Here's how the part is built. I have some questions about the finished solid (model axes, mm). A direction names the side the tool comes from. Coordinates: 2 decimals unless noted, no trailing zeros. Loops run counter-clockwise (first coordinate to the right, second up) from the corner with the lowest first, then second, coordinate; pieces in that order, holes last. Notation, with made-up numbers: (19, -30) -> (66, -30) arc R29 cw to (66, -10) -> close; hole circle Ø6 at (73, -27.75). An arc over 180 degrees is marked (long way). Answer as a JSON object with one key per item and string values. Group by question number.
1) If we mould it in two halves opening along Z, with no side actions, what happens to faces 1 (the flat face through (-1, 3, -6)), 2 (the cylindrical face through (62.325, 1.479, 108.237)), 3 (the cylindrical face through (48.55, 1.52, 68.16))? For each: +Z half, -Z half, draft (parallel to the pull), parting line (faces both ways), or undercut.
2) I need wall thicknesses on probe 1 along Z at (x, y) = (-31, 1.4); probe 2 along X at (y, z) = (1, -110); probe 3 along Z at (x, y) = (-54, 2.35). Which ranges of each line are inside material? Lowest first, please. Write a range as [from, to].
3) I want a section at C-C (y = 1.55). Count the separate pieces of the cut face and the enclosed holes in it, then the cut area to 3 significant figures.
4) I want a section at A-A (x = 23.5). Write out the boundary of the cut face in (y, z).
5) I want a section at B-B (x = 6.5). Write out the boundary of the cut face in (y, z), then the cut area to 3 significant figures.
6) I'm going to push flat-ended pins straight in: pin 1 (2 mm diameter, centred on x = 14.5, z = 67.27, fed in from +Y); pin 2 (3 mm diameter, centred on x = -34.5, z = 86.5, fed in from -Y); pin 3 (1.6 mm diameter, centred on x = 34.5, y = 1.5, fed in from +Z). Where does each tip first touch, or does it pass through?
7) Which directions (+Z, -Z, +X, -X, +Y, -Y) give clear straight access to the entire face, cutting with the end or side of a thin tool? Please do faces 4 (the cylindrical face through (-62.325, 1.479, 108.237)), 5 (the cylindrical face through (56.1, 1.5, 34.4)), 6 (the cylindrical face through (-41.32, 1.48, 108.24)).
```python
from build123d import *

# Parameters (mm, degrees)
SKETCH1_W           = 180
SKETCH1_H           = 240
BOSS_EXTRUDE1_DEPTH = 3
SKETCH3_R           = 1.55
CUT_EXTRUDE2_DEPTH  = 151.029997001
SKETCH4_R           = 1.6
SKETCH4_R_2         = 1.65
CUT_EXTRUDE3_DEPTH  = 151.029997001
SKETCH5_R           = 1.6
CUT_EXTRUDE4_DEPTH  = 151.029997001
SKETCH6_R           = 1.55
CUT_EXTRUDE5_DEPTH  = 151.029997001
SKETCH7_W           = 25.678556749
SKETCH7_H           = 240
SKETCH7_W_2         = 78.7
SKETCH7_H_2         = 25
CUT_EXTRUDE6_DEPTH  = 151.029997001
SKETCH8_W           = 128.642886502
SKETCH8_H           = 9.657988802
CUT_EXTRUDE7_DEPTH  = 137.184610224
FILLET1_R           = 7


with BuildPart() as part:
    # Sketch1 → Boss-Extrude1 (new body)
    with BuildSketch(Plane(origin=(0, 0, 0), x_dir=(1, 0, 0), z_dir=(0, 1, 0))):
        Rectangle(SKETCH1_W, SKETCH1_H)
    extrude(amount=BOSS_EXTRUDE1_DEPTH)

    # Sketch3 → Cut-Extrude2 (cut, through all)
    with BuildSketch(Plane(origin=(0, 3, 0), x_dir=(1, 0, 0), z_dir=(0, 1, 0))):
        with Locations(Location((14, 110, 0), (0, 0, 270))):
            Circle(SKETCH3_R)
        with Locations(Location((-14, 110, 0), (0, 0, 90))):
            Circle(SKETCH3_R)
    extrude(amount=-CUT_EXTRUDE2_DEPTH, mode=Mode.SUBTRACT)

    # Sketch4 → Cut-Extrude3 (cut, through all)
    with BuildSketch(Plane(origin=(0, 3, 0), x_dir=(1, 0, 0), z_dir=(0, 1, 0))):
        with Locations(Location((-50.5, -32.268683434, 0), (0, 0, 270))):
            Circle(SKETCH4_R)
        with Locations(Location((-50.5, -67.268683434, 0), (0, 0, 270))):
            Circle(SKETCH4_R)
        with Locations(Location((14.5, -32.268683434, 0), (0, 0, 270))):
            Circle(SKETCH4_R_2)
        with Locations(Location((14.5, -67.268683434, 0), (0, 0, 270))):
            Circle(SKETCH4_R_2)
    extrude(amount=-CUT_EXTRUDE3_DEPTH, mode=Mode.SUBTRACT)

    # Sketch5 → Cut-Extrude4 (cut, through all)
    with BuildSketch(Plane(origin=(0, 3, 0), x_dir=(1, 0, 0), z_dir=(0, 1, 0))):
        with Locations(Location((56, 54.660722259, 0), (0, 0, 270))):
            Circle(SKETCH5_R)
        with Locations(Location((56, -18.339277741, 0), (0, 0, 270))):
            Circle(SKETCH5_R)
        with Locations(Location((-56, -18.339277741, 0), (0, 0, 270))):
            Circle(SKETCH5_R)
        with Locations(Location((-56, 54.660722259, 0), (0, 0, 270))):
            Circle(SKETCH5_R)
    extrude(amount=-CUT_EXTRUDE4_DEPTH, mode=Mode.SUBTRACT)

    # Sketch6 → Cut-Extrude5 (cut, through all)
    with BuildSketch(Plane(origin=(0, 3, 0), x_dir=(1, 0, 0), z_dir=(0, 1, 0))):
        with Locations(Location((-54.321443251, -103.342011198, 0), (0, 0, 270))):
            Circle(SKETCH6_R)
        with Locations(Location((54.378556749, -103.342011198, 0), (0, 0, 270))):
            Circle(SKETCH6_R)
        with Locations(Location((-54.321443251, 104.657988802, 0), (0, 0, 270))):
            Circle(SKETCH6_R)
        with Locations(Location((54.378556749, 104.657988802, 0), (0, 0, 270))):
            Circle(SKETCH6_R)
    extrude(amount=-CUT_EXTRUDE5_DEPTH, mode=Mode.SUBTRACT)

    # Sketch7 → Cut-Extrude6 (cut, through all)
    with BuildSketch(Plane(origin=(0, 3, 0), x_dir=(1, 0, 0), z_dir=(0, 1, 0))):
        with BuildLine():
            Line((37.630016224, 79.701073582), (12.399273995, 79.701073582))
            ThreePointArc((12.399273995, 79.701073582), (10.985060433, 80.286860019), (10.399273995, 81.701073582))
            Line((10.399273995, 81.701073582), (10.399273995, 81.912178755))
            ThreePointArc((10.399273995, 81.912178755), (10.985060433, 83.326392317), (12.399273995, 83.912178755))
            Line((12.399273995, 83.912178755), (37.630016224, 83.912178755))
            ThreePointArc((37.630016224, 83.912178755), (39.044229786, 83.326392317), (39.630016224, 81.912178755))
            Line((39.630016224, 81.912178755), (39.630016224, 81.701073582))
            ThreePointArc((39.630016224, 81.701073582), (39.044229786, 80.286860019), (37.630016224, 79.701073582))
        make_face()
        with BuildLine():
            Line((-37.630016224, 83.912178755), (-12.399273995, 83.912178755))
            ThreePointArc((-12.399273995, 83.912178755), (-10.985060433, 83.326392317), (-10.399273995, 81.912178755))
            Line((-10.399273995, 81.912178755), (-10.399273995, 81.701073582))
            ThreePointArc((-10.399273995, 81.701073582), (-10.985060433, 80.286860019), (-12.399273995, 79.701073582))
            Line((-12.399273995, 79.701073582), (-37.630016224, 79.701073582))
            ThreePointArc((-37.630016224, 79.701073582), (-39.044229786, 80.286860019), (-39.630016224, 81.701073582))
            Line((-39.630016224, 81.701073582), (-39.630016224, 81.912178755))
            ThreePointArc((-39.630016224, 81.912178755), (-39.044229786, 83.326392317), (-37.630016224, 83.912178755))
        make_face()
        with Locations((-77.160721626, 0)):
            Rectangle(SKETCH7_W, SKETCH7_H)
        with Locations((0.028556749, -107.5)):
            Rectangle(SKETCH7_W_2, SKETCH7_H_2)
        with Locations((77.160721626, 0)):
            Rectangle(SKETCH7_W, SKETCH7_H)
        with BuildLine():
            Line((29.345445331, -37.30118784), (29.345445331, -65.30118784))
            ThreePointArc((29.345445331, -65.30118784), (30.517018206, -68.129614965), (33.345445331, -69.30118784))
            Line((33.345445331, -69.30118784), (35.345445331, -69.30118784))
            ThreePointArc((35.345445331, -69.30118784), (38.173872456, -68.129614965), (39.345445331, -65.30118784))
            Line((39.345445331, -65.30118784), (39.345445331, -37.30118784))
            ThreePointArc((39.345445331, -37.30118784), (38.173872456, -34.472760715), (35.345445331, -33.30118784))
            Line((35.345445331, -33.30118784), (33.345445331, -33.30118784))
            ThreePointArc((33.345445331, -33.30118784), (30.517018206, -34.472760715), (29.345445331, -37.30118784))
        make_face()
        with BuildLine():
            Line((51.345445331, -33.30118784), (53.345445331, -33.30118784))
            ThreePointArc((53.345445331, -33.30118784), (56.173872456, -34.472760715), (57.345445331, -37.30118784))
            Line((57.345445331, -37.30118784), (57.345445331, -65.30118784))
            ThreePointArc((57.345445331, -65.30118784), (56.173872456, -68.129614965), (53.345445331, -69.30118784))
            Line((53.345445331, -69.30118784), (51.345445331, -69.30118784))
            ThreePointArc((51.345445331, -69.30118784), (48.517018206, -68.129614965), (47.345445331, -65.30118784))
            Line((47.345445331, -65.30118784), (47.345445331, -37.30118784))
            ThreePointArc((47.345445331, -37.30118784), (48.517018206, -34.472760715), (51.345445331, -33.30118784))
        make_face()
        with BuildLine():
            Line((37.630016224, 94.701073582), (12.399273995, 94.701073582))
            ThreePointArc((12.399273995, 94.701073582), (10.985060433, 95.286860019), (10.399273995, 96.701073582))
            Line((10.399273995, 96.701073582), (10.399273995, 96.912178755))
            ThreePointArc((10.399273995, 96.912178755), (10.985060433, 98.326392317), (12.399273995, 98.912178755))
            Line((12.399273995, 98.912178755), (37.630016224, 98.912178755))
            ThreePointArc((37.630016224, 98.912178755), (39.044229786, 98.326392317), (39.630016224, 96.912178755))
            Line((39.630016224, 96.912178755), (39.630016224, 96.701073582))
            ThreePointArc((39.630016224, 96.701073582), (39.044229786, 95.286860019), (37.630016224, 94.701073582))
        make_face()
        with BuildLine():
            Line((-37.630016224, 98.912178755), (-12.399273995, 98.912178755))
            ThreePointArc((-12.399273995, 98.912178755), (-10.985060433, 98.326392317), (-10.399273995, 96.912178755))
            Line((-10.399273995, 96.912178755), (-10.399273995, 96.701073582))
            ThreePointArc((-10.399273995, 96.701073582), (-10.985060433, 95.286860019), (-12.399273995, 94.701073582))
            Line((-12.399273995, 94.701073582), (-37.630016224, 94.701073582))
            ThreePointArc((-37.630016224, 94.701073582), (-39.044229786, 95.286860019), (-39.630016224, 96.701073582))
            Line((-39.630016224, 96.701073582), (-39.630016224, 96.912178755))
            ThreePointArc((-39.630016224, 96.912178755), (-39.044229786, 98.326392317), (-37.630016224, 98.912178755))
        make_face()
    extrude(amount=-CUT_EXTRUDE6_DEPTH, mode=Mode.SUBTRACT)

    # Sketch8 → Cut-Extrude7 (cut, through all)
    with BuildSketch(Plane(origin=(0, 3, 0), x_dir=(1, 0, 0), z_dir=(0, 1, 0))):
        with Locations((0, -115.171005599)):
            Rectangle(SKETCH8_W, SKETCH8_H)
    extrude(amount=-CUT_EXTRUDE7_DEPTH, mode=Mode.SUBTRACT)

    # Fillet1
    fillet1_edges = [part.edges().sort_by_distance(p)[0] for p in [
        (-64.321443251, 1.5, -120),
        (-39.321443251, 1.5, 95),
        (39.378556749, 1.5, 95),
        (64.321443251, 1.5, -120),
        (39.378556749, 1.5, 110.342011198),
        (-39.321443251, 1.5, 110.342011198),
        (-64.321443251, 1.5, 110.342011198),
        (64.321443251, 1.5, 110.342011198),
    ]]
    fillet(fillet1_edges, radius=FILLET1_R)


solid = part.part
```
Determined:
{
 "1": {"face 1": "draft", "face 2": "+Z half", "face 3": "undercut"},
 "2": {"probe 1": "[-120, -98.91], [-94.7, -83.91], [-79.7, 95]", "probe 2": "[-64.32, -15.55], [-12.45, 12.45], [15.55, 64.32]", "probe 3": "[-120, -106.17], [-103.14, 101.83], [104.86, 110.34]"},
 "3": {"separate pieces": "1", "enclosed holes": "20", "area": "27,100 mm^2"},
 "4": {"outline": "(0, -120) -> (3, -120) -> (3, -98.91) -> (0, -98.91) -> close; (0, -94.7) -> (3, -94.7) -> (3, -83.91) -> (0, -83.91) -> close; (0, -79.7) -> (3, -79.7) -> (3, 95) -> (0, 95) -> close"},
 "5": {"outline": "(0, -120) -> (3, -120) -> (3, 95) -> (0, 95) -> close", "area": "645 mm^2"},
 "6": {"pin 1": "through", "pin 2": "y = 0", "pin 3": "z = 95.64"},
 "7": {"face 4": "+Z, -X, +Y, -Y", "face 5": "+Y, -Y", "face 6": "+Z, +Y, -Y"}
}
